Autodesk Inventor part; units mm, degrees
ref_plane "YZ Plane" through (0, 0, 0) normal (1, 0, 0) x (0, 1, 0)
ref_plane "XZ Plane" through (0, 0, 0) normal (0, 1, 0) x (-1, 0, 0)
ref_plane "XY Plane" through (0, 0, 0) normal (0, 0, 1) x (1, 0, 0)
sketch "Sketch1" plane through (0, 0, 0) normal (0, 0, 1) x (1, 0, 0)
  line L0 (0, 0) -> (-225, 0)
  line L1 (-225, 0) -> (-225, 45)
  line L2 (-225, 45) -> (0, 45)
  line L3 (0, 45) -> (0, 0)
  circle A0 centre (-10, 37.5) radius 1.5
  circle A1 centre (-10, 7.5) radius 1.5
  circle A2 centre (-214.479, 37.5) radius 1.5
  circle A3 centre (-215, 7.5) radius 1.5
  circle A4 centre (-109.8876, 25.0816) radius 4.5358
  circle A5 centre (-170.8457, 21.6854) radius 5.3121
  circle A6 centre (-54.5027, 21.6854) radius 5.3121
  dimension "d0" = 45
  dimension "d1" = 225
  dimension "d2" = 30
  dimension "d3" = 3
  dimension "d4" = 3
  dimension "d5" = 7.5
  dimension "d6" = 7.5
  dimension "d7" = 3
  dimension "d8" = 3
  dimension "d9" = 30
  dimension "d10" = 10
  dimension "d11" = 10
extrude "Extrusion1" add sketch "Sketch1" along normal blind 10
equation "\"d6\" = d5"
equation "\"d7\" = d4"
equation "\"d8\" = d7"
equation "\"d9\" = d2"
properties part number "PlateHeatbed"
For this review, take the finished solid that the model builds, in its own axes (mm). Coordinates: 2 decimals unless noted, no trailing zeros. Use CSV: the item, a comma, the result in double quotes. Start each with the question number.
Item 1: Draft analysis for pull direction X (two halves, no side actions). For faces 1 (the face through (-114, 45, 5)), 2 (the face through (-225, 22, 5)), 3 (the face through (-105.7, 26.82, 4.93)), state which applies: pulls with the +X half, pulls with the -X half, needs draft (parallel to the pull), parting line crosses it, or undercut.
Item 2: Insertion check: pin 1 (10.5 mm diameter, centred on x = -109.89, y = 25.08, fed in from -Z). The pin has a flat end and moves straight along its axis. Give the tip position at first contact, or say it passes through.
Item 3: Wall thickness on probe 1 along Y at (x, z) = (-10, 6); probe 2 along X at (y, z) = (26.5, 1); probe 3 along X at (y, z) = (24, 2.25): over which ranges is each line inside the solid? List them lowest first.
Derived:
1,face 1,"needs draft"
1,face 2,"pulls with the -X half"
1,face 3,"undercut"
2,pin 1,"stops at z = 0"
3,probe 1,"y = 0 to 6, 9 to 36, 39 to 45"
3,probe 2,"x = -225 to -173.09, -168.6 to -114.2, -105.58 to -56.75, -52.26 to 0"
3,probe 3,"x = -225 to -175.63, -166.06 to -114.29, -105.48 to -59.28, -49.72 to 0"
